Here's the drawing with two shaded views (mm, measured from the low corner). I have some questions. A direction names the side the tool comes from. Coordinates: 2 decimals unless noted, no trailing zeros. Order: outer loops, then holes, each group sorted by start corner. A loop starts at its lowest first (then second) coordinate and runs counter-clockwise, first axis right, second up. Notation, with made-up numbers: M 89,-36 L 135,-36 A14 cw 135,-15 Z; hole C 67,7 d6. An arc over 180 degrees is marked long. Put each result on its own line as item: value. Start each with the question number.
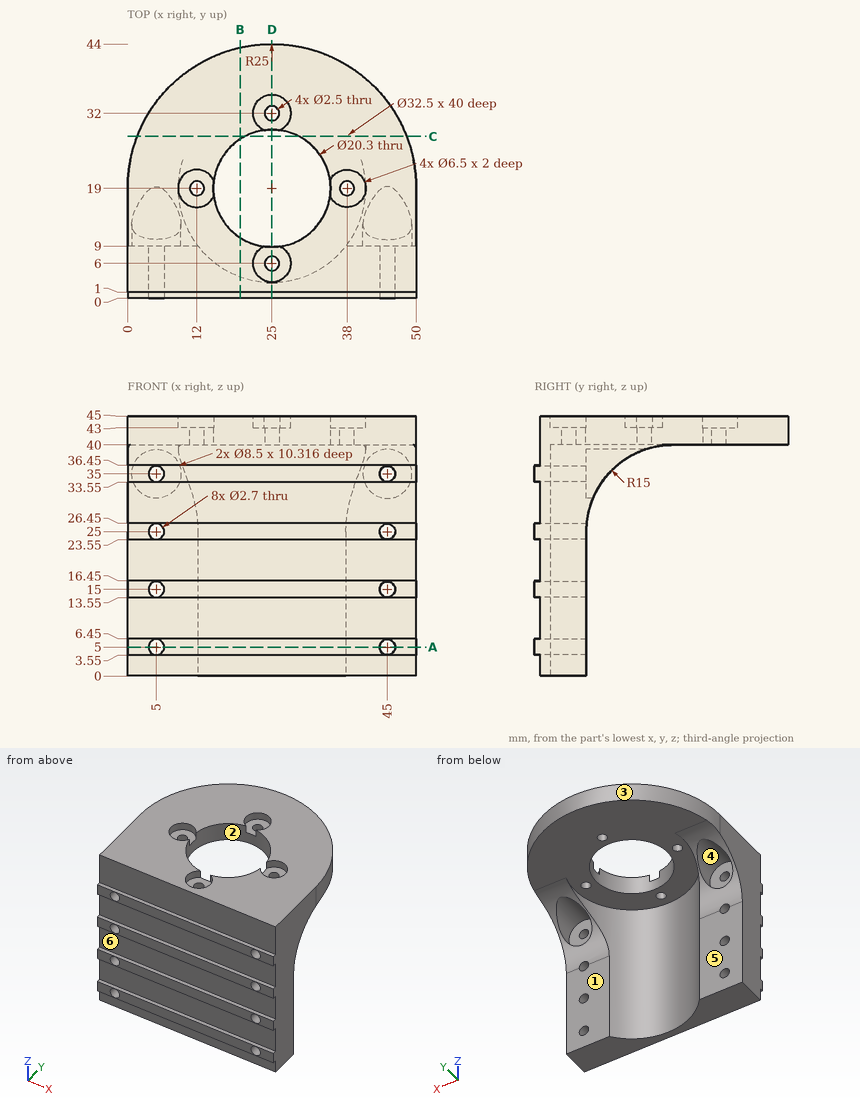
Item 1: If we mould it in two halves opening along X, with no side actions, what happens to the marked faces 1, 2 and 3? For each: released by +X, released by -X, zero draft, split by the parting line, or undercut.
Item 2: If we section it at C-C on y = 28: Write out the boundary of the cut face in (x, z), then the cut area to 3 significant figures.
Item 3: For the marked faces 4, 5 and 6, which set-ups out of +Z, -Z, +X, -X, +Y, -Y let a thin tool reach every point of the face, with its end or its side?
Item 4: If we section it at A-A on z = 5: Write out the boundary of the cut face in (x, y), then the cut area to 3 significant figures.
Item 5: If we section it at D-D on x = 25: State how many separate pieces and enclosed holes the cut face has, then the cut area to 3 significant figures.
Item 6: I need wall thicknesses on probe 1 along Y at (x, z) = (25, 42); probe 2 along Z at (x, y) = (21, 34); probe 3 along X at (y, z) = (5, 43.5). Which ranges of each line are inside material? Lowest first, please.
Item 7: For pin 1 Ø2 at (x, z) = (24, 12) entering from -Y; pin 2 Ø4.5 at (x, z) = (5, 5) entering from +Y; pin 3 Ø2.5 at (x, z) = (5, 35) entering from -Y; pin 4 Ø5 at (x, y) = (37, 20) entering from +Z, each with a flat end and sliding along its axis, tell me the tip position at first contact or that it passes through.
Item 8: If we section it at B-B on x = 19.5: Write out the boundary of the cut face in (y, z).
Geometry check:
1. face 1: zero draft
1. face 2: undercut
1. face 3: split by the parting line
2. outline: M 1.68,40 L 20.31,40 L 20.31,45 L 1.68,45 Z; M 29.69,40 L 48.32,40 L 48.32,45 L 29.69,45 Z
2. area: 186 mm²
3. face 4: +Y
3. face 5: -Z, +X, -X, +Y
3. face 6: +X, -X, -Y
4. outline: M 0,0 L 3.65,0 L 3.65,9 L 0,9 Z; M 6.35,0 L 43.65,0 L 43.65,9 L 37.81,9 A16.25 cw 12.19,9 L 6.35,9 Z; M 46.35,0 L 50,0 L 50,9 L 46.35,9 Z
4. area: 290 mm²
5. separate pieces: 4
5. enclosed holes: 0
5. area: 156 mm²
6. probe 1: y = 1 to 4.75, 7.25 to 8.85, 29.15 to 30.75, 33.25 to 44
6. probe 2: z = 40 to 45
6. probe 3: x = 0 to 21.91, 28.09 to 50
7. pin 1: stops at y = 1
7. pin 2: stops at y = 9
7. pin 3: passes through
7. pin 4: stops at z = 45
8. outline: M 0,3.55 L 1,3.55 L 1,0 L 3.71,0 L 3.71,40 L 10.47,40 L 10.47,45 L 1,45 L 1,36.45 L 0,36.45 L 0,33.55 L 1,33.55 L 1,26.45 L 0,26.45 L 0,23.55 L 1,23.55 L 1,16.45 L 0,16.45 L 0,13.55 L 1,13.55 L 1,6.45 L 0,6.45 Z; M 27.53,40 L 43.39,40 L 43.39,45 L 27.53,45 Z
